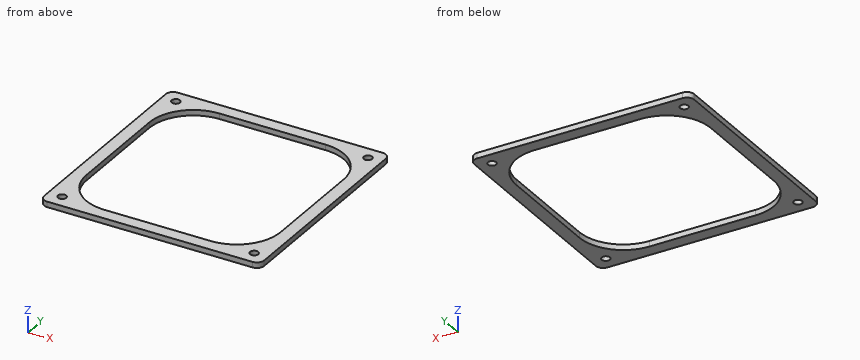
Autodesk Inventor part; units mm, degrees
ref_plane "YZ Plane" through (0, 0, 0) normal (1, 0, 0) x (0, 1, 0)
ref_plane "XZ Plane" through (0, 0, 0) normal (0, 1, 0) x (-1, 0, 0)
ref_plane "XY Plane" through (0, 0, 0) normal (0, 0, 1) x (1, 0, 0)
sketch "スケッチ1" plane through (0, 0, 0) normal (0, 0, 1) x (1, 0, 0)
  circle A0 centre (5, 125) radius 2.25 construction
  circle A1 centre (5, 5) radius 2.25 construction
  circle A2 centre (-473, 125) radius 2.25 construction
  circle A3 centre (-473, 5) radius 2.25 construction
  line L0 (-478, 130) -> (-478, 0) construction
  line L1 (10, 0) -> (10, 130) construction
  line L2 (10, 130) -> (-478, 130)
  line L3 (-478, 130) -> (-478, 0)
  line L4 (-478, 0) -> (10, 0)
  line L5 (10, 0) -> (10, 130)
  circle A4 centre (5, 125) radius 1.6
  circle A5 centre (5, 5) radius 1.6
  circle A6 centre (-473, 5) radius 1.6
  circle A7 centre (-473, 125) radius 1.6
  line L6 (10, 65) -> (-478, 65) construction
  line L7 (-205, 118) -> (-263, 118)
  line L8 (-287, 94) -> (-287, 36)
  line L9 (-263, 12) -> (-205, 12)
  line L10 (-181, 36) -> (-181, 94)
  arc A8 (-181, 94) -> (-205, 118) centre (-205, 94) ccw
  arc A9 (-205, 12) -> (-181, 36) centre (-205, 36) ccw
  arc A10 (-287, 36) -> (-263, 12) centre (-263, 36) ccw
  arc A11 (-263, 118) -> (-287, 94) centre (-263, 94) ccw
  line L11 (-174, 125) -> (-294, 125) construction
  line L12 (-294, 125) -> (-294, 5) construction
  line L13 (-294, 5) -> (-174, 5) construction
  line L14 (-174, 5) -> (-174, 125) construction
  line L15 (-181.6, 117.4) -> (-286.4, 117.4) construction
  line L16 (-286.4, 117.4) -> (-286.4, 12.6) construction
  line L17 (-286.4, 12.6) -> (-181.6, 12.6) construction
  line L18 (-181.6, 12.6) -> (-181.6, 117.4) construction
  circle A12 centre (-181.6, 117.4) radius 2.25
  circle A13 centre (-181.6, 12.6) radius 2.25
  circle A14 centre (-286.4, 12.6) radius 2.25
  circle A15 centre (-286.4, 117.4) radius 2.25
  circle A16 centre (-301.6, 117.4) radius 2.25
  arc A17 (-301, 94) -> (-325, 118) centre (-325, 94) ccw
  line L19 (-301, 36) -> (-301, 94)
  arc A18 (-325, 12) -> (-301, 36) centre (-325, 36) ccw
  circle A19 centre (-301.6, 12.6) radius 2.25
  line L20 (-383, 12) -> (-325, 12)
  arc A20 (-407, 36) -> (-383, 12) centre (-383, 36) ccw
  circle A21 centre (-406.4, 12.6) radius 2.25
  line L21 (-407, 94) -> (-407, 36)
  circle A22 centre (-406.4, 117.4) radius 2.25
  arc A23 (-383, 118) -> (-407, 94) centre (-383, 94) ccw
  line L22 (-325, 118) -> (-383, 118)
  circle A24 centre (-61.6, 117.4) radius 2.25
  arc A25 (-61, 94) -> (-85, 118) centre (-85, 94) ccw
  line L23 (-61, 36) -> (-61, 94)
  arc A26 (-85, 12) -> (-61, 36) centre (-85, 36) ccw
  circle A27 centre (-61.6, 12.6) radius 2.25
  line L24 (-143, 12) -> (-85, 12)
  arc A28 (-167, 36) -> (-143, 12) centre (-143, 36) ccw
  circle A29 centre (-166.4, 12.6) radius 2.25
  line L25 (-167, 94) -> (-167, 36)
  circle A30 centre (-166.4, 117.4) radius 2.25
  arc A31 (-143, 118) -> (-167, 94) centre (-143, 94) ccw
  line L26 (-85, 118) -> (-143, 118)
  circle A32 centre (-181.6, 117.4) radius 2.25
  arc A33 (-181, 94) -> (-205, 118) centre (-205, 94) ccw
  line L27 (-181, 36) -> (-181, 94)
  arc A34 (-205, 12) -> (-181, 36) centre (-205, 36) ccw
  circle A35 centre (-181.6, 12.6) radius 2.25
  line L28 (-263, 12) -> (-205, 12)
  arc A36 (-287, 36) -> (-263, 12) centre (-263, 36) ccw
  circle A37 centre (-286.4, 12.6) radius 2.25
  line L29 (-287, 94) -> (-287, 36)
  circle A38 centre (-286.4, 117.4) radius 2.25
  arc A39 (-263, 118) -> (-287, 94) centre (-263, 94) ccw
  line L30 (-205, 118) -> (-263, 118)
  point P0 (0, 0)
  point P1 (-234, 65)
  point P2 (-287, 12)
  point P3 (-287, 118)
  point P4 (-181, 12)
  point P5 (-287, 65)
  point P6 (-294, 65)
  point P7 (-234, 12)
  point P8 (-234, 5)
  point P9 (-234, 118)
  point P10 (-181, 65)
  point P11 (-174, 65)
  point P12 (-181.6, 65)
  point P13 (-234, 125)
  point P14 (-234, 117.4)
  point P15 (-301, 12)
  point P16 (-301, 65)
  point P17 (-407, 12)
  point P18 (-354, 12)
  point P19 (-407, 118)
  point P20 (-407, 65)
  point P21 (-354, 118)
  point P22 (-61, 12)
  point P23 (-61, 65)
  point P24 (-167, 12)
  point P25 (-114, 12)
  point P26 (-167, 118)
  point P27 (-167, 65)
  point P28 (-114, 118)
  point P29 (-181, 12)
  point P30 (-181, 65)
  point P31 (-287, 12)
  point P32 (-234, 12)
  point P33 (-287, 118)
  point P34 (-287, 65)
  point P35 (-234, 118)
  dimension "d0" = 3.2
  dimension "d1" = 106
  dimension "d2" = 106
  dimension "d3" = 24
  dimension "d4" = 120
  dimension "d5" = 120
  dimension "d6" = 104.8
  dimension "d7" = 104.8
  dimension "d8" = 4.5
  dimension "d11" = 120
  dimension "d14" = 120
extrude "押し出し1" add sketch "スケッチ1" along normal blind 3
sketch "スケッチ2" plane through (0, 0, 3) normal (0, 0, 1) x (1, 0, 0)
  line L0 (-478, 130) -> (-478, 0)
  line L1 (-478, 0) -> (10, 0)
  line L2 (10, 0) -> (10, 130)
  line L3 (10, 130) -> (-478, 130)
  circle A0 centre (-286.4, 117.4) radius 2.25
  arc A1 (-263, 118) -> (-287, 94) centre (-263, 94) ccw
  line L4 (-263, 118) -> (-205, 118)
  arc A2 (-181, 94) -> (-205, 118) centre (-205, 94) ccw
  line L5 (-181, 94) -> (-181, 36)
  arc A3 (-205, 12) -> (-181, 36) centre (-205, 36) ccw
  line L6 (-205, 12) -> (-263, 12)
  arc A4 (-287, 36) -> (-263, 12) centre (-263, 36) ccw
  line L7 (-287, 36) -> (-287, 94)
  circle A5 centre (-473, 125) radius 1.6
  circle A6 centre (-473, 5) radius 1.6
  circle A7 centre (5, 5) radius 1.6
  circle A8 centre (5, 125) radius 1.6
  circle A9 centre (-181.6, 117.4) radius 2.25
  circle A10 centre (-181.6, 12.6) radius 2.25
  circle A11 centre (-286.4, 12.6) radius 2.25
  circle A12 centre (-166.4, 117.4) radius 2.25
  circle A13 centre (-166.4, 12.6) radius 2.25
  circle A14 centre (-61.6, 12.6) radius 2.25
  line L8 (-61, 94) -> (-61, 36)
  arc A15 (-85, 12) -> (-61, 36) centre (-85, 36) ccw
  line L9 (-85, 12) -> (-143, 12)
  arc A16 (-167, 36) -> (-143, 12) centre (-143, 36) ccw
  line L10 (-167, 36) -> (-167, 94)
  arc A17 (-143, 118) -> (-167, 94) centre (-143, 94) ccw
  line L11 (-143, 118) -> (-85, 118)
  arc A18 (-61, 94) -> (-85, 118) centre (-85, 94) ccw
  circle A19 centre (-61.6, 117.4) radius 2.25
  circle A20 centre (-406.4, 117.4) radius 2.25
  circle A21 centre (-406.4, 12.6) radius 2.25
  circle A22 centre (-301.6, 12.6) radius 2.25
  line L12 (-301, 94) -> (-301, 36)
  arc A23 (-325, 12) -> (-301, 36) centre (-325, 36) ccw
  line L13 (-325, 12) -> (-383, 12)
  arc A24 (-407, 36) -> (-383, 12) centre (-383, 36) ccw
  line L14 (-407, 36) -> (-407, 94)
  arc A25 (-383, 118) -> (-407, 94) centre (-383, 94) ccw
  line L15 (-383, 118) -> (-325, 118)
  arc A26 (-301, 94) -> (-325, 118) centre (-325, 94) ccw
  circle A27 centre (-301.6, 117.4) radius 2.25
  line L16 (-477.9, 129.9) -> (-477.9, 0.1)
  line L17 (-477.9, 0.1) -> (9.9, 0.1)
  line L18 (9.9, 0.1) -> (9.9, 129.9)
  line L19 (9.9, 129.9) -> (-477.9, 129.9)
  point P0 (0, 0)
  dimension "d19" = 0.1
extrude "押し出し2" cut sketch "スケッチ2" against normal through all contours L3 L2 L1 L0
fillet "フィレット1" radius 2 4 edges at (-477.9, 129.9, 1.5) (-477.9, 0.1, 1.5) (9.9, 0.1, 1.5) (9.9, 129.9, 1.5)
sketch "スケッチ3" plane through (0, 0, 3) normal (0, 0, 1) x (1, 0, 0)
  arc A0 (9.9, 127.9) -> (7.9, 129.9) centre (7.9, 127.9) ccw
  line L0 (7.9, 129.9) -> (-475.9, 129.9)
  arc A1 (-475.9, 129.9) -> (-477.9, 127.9) centre (-475.9, 127.9) ccw
  line L1 (-477.9, 127.9) -> (-477.9, 2.1)
  arc A2 (-477.9, 2.1) -> (-475.9, 0.1) centre (-475.9, 2.1) ccw
  line L2 (-475.9, 0.1) -> (7.9, 0.1)
  arc A3 (7.9, 0.1) -> (9.9, 2.1) centre (7.9, 2.1) ccw
  line L3 (9.9, 2.1) -> (9.9, 127.9)
  circle A4 centre (-286.4, 117.4) radius 2.25
  arc A5 (-263, 118) -> (-287, 94) centre (-263, 94) ccw
  line L4 (-263, 118) -> (-205, 118)
  arc A6 (-181, 94) -> (-205, 118) centre (-205, 94) ccw
  line L5 (-181, 94) -> (-181, 36)
  arc A7 (-205, 12) -> (-181, 36) centre (-205, 36) ccw
  line L6 (-205, 12) -> (-263, 12)
  arc A8 (-287, 36) -> (-263, 12) centre (-263, 36) ccw
  line L7 (-287, 36) -> (-287, 94)
  circle A9 centre (-473, 125) radius 1.6
  circle A10 centre (-473, 5) radius 1.6
  circle A11 centre (5, 5) radius 1.6
  circle A12 centre (5, 125) radius 1.6
  circle A13 centre (-181.6, 117.4) radius 2.25
  circle A14 centre (-181.6, 12.6) radius 2.25
  circle A15 centre (-286.4, 12.6) radius 2.25
  circle A16 centre (-166.4, 117.4) radius 2.25
  circle A17 centre (-166.4, 12.6) radius 2.25
  circle A18 centre (-61.6, 12.6) radius 2.25
  line L8 (-61, 94) -> (-61, 36)
  arc A19 (-85, 12) -> (-61, 36) centre (-85, 36) ccw
  line L9 (-85, 12) -> (-143, 12)
  arc A20 (-167, 36) -> (-143, 12) centre (-143, 36) ccw
  line L10 (-167, 36) -> (-167, 94)
  arc A21 (-143, 118) -> (-167, 94) centre (-143, 94) ccw
  line L11 (-143, 118) -> (-85, 118)
  arc A22 (-61, 94) -> (-85, 118) centre (-85, 94) ccw
  circle A23 centre (-61.6, 117.4) radius 2.25
  circle A24 centre (-406.4, 117.4) radius 2.25
  circle A25 centre (-406.4, 12.6) radius 2.25
  circle A26 centre (-301.6, 12.6) radius 2.25
  line L12 (-301, 94) -> (-301, 36)
  arc A27 (-325, 12) -> (-301, 36) centre (-325, 36) ccw
  line L13 (-325, 12) -> (-383, 12)
  arc A28 (-407, 36) -> (-383, 12) centre (-383, 36) ccw
  line L14 (-407, 36) -> (-407, 94)
  arc A29 (-383, 118) -> (-407, 94) centre (-383, 94) ccw
  line L15 (-383, 118) -> (-325, 118)
  arc A30 (-301, 94) -> (-325, 118) centre (-325, 94) ccw
  circle A31 centre (-301.6, 117.4) radius 2.25
  line L16 (-410, 125) -> (-58, 125)
  line L17 (-54, 121) -> (-54, 9)
  line L18 (-58, 5) -> (-410, 5)
  line L19 (-414, 9) -> (-414, 121)
  arc A32 (-410, 125) -> (-414, 121) centre (-410, 121) ccw
  arc A33 (-414, 9) -> (-410, 5) centre (-410, 9) ccw
  arc A34 (-58, 5) -> (-54, 9) centre (-58, 9) ccw
  arc A35 (-54, 121) -> (-58, 125) centre (-58, 121) ccw
  line L20 (-294, 125) -> (-294, 5)
  point P0 (0, 0)
  point P1 (-414, 125)
  point P2 (-54, 125)
  point P3 (-234, 125)
  point P4 (-234, 118)
  point P5 (-414, 65)
  point P6 (-407, 65)
  dimension "d23" = 120
  dimension "d24" = 360
  dimension "d25" = 4
  dimension "d28" = 120
extrude "押し出し3" cut sketch "スケッチ3" against normal blind 10 contours A24 | A25 | A26 | A31 | L16 L20 L18 A33 L19 A32 keep common part
fillet "フィレット2" radius 4 2 edges at (-294, 125, 1.5) (-294, 5, 1.5)
equation "\"d5\" = d4"
equation "\"d7\" = d6"
properties part number "radiator_adapter_04"
The listing builds one solid part. Answer for the finished solid, in the listing's coordinates (mm). Give positions to 0.01 mm unless a question says otherwise; leave off trailing zeros. Write each loop counter-clockwise with the first axis right and the second up, starting at its lowest first coordinate (ties: lowest second). Pieces come first, ordered by that corner, then holes. Notation, with made-up numbers: (79, 32) - (136, 32) arc R20 cw to (136, 51) - close; hole circle Ø11 at (46.25, 46). An arc over 180 degrees is marked (long way). Use one line per item in the form item = value. Start each with the question number.
1) Find section C-C on z = 2.1. Determine the outline of the cut face in (x, y), plus the area to 3 significant figures.
2) Find section A-A on x = -343. Determine the outline of the cut face in (y, z).
3) Find section B-B on y = 91. Determine the outline of the cut face in (x, z), plus the area to 3 significant figures.
4) Consider line 1 along Y through (x, z) = (-353, 1.1); line 2 along X through (y, z) = (45, 1); line 3 along X through (y, z) = (105, 1.1). Determine where each line is inside the solid, lowest interval first. Write a range as from..to.
Geometry results:
q1.outline = (-414, 9) arc R4 ccw to (-410, 5) - (-298, 5) arc R4 ccw to (-294, 9) - (-294, 121) arc R4 ccw to (-298, 125) - (-410, 125) arc R4 ccw to (-414, 121) - close; hole circle Ø4.5 at (-406.4, 12.6); hole circle Ø4.5 at (-406.4, 117.4); hole (-407, 36) arc R24 ccw to (-383, 12) - (-325, 12) arc R24 ccw to (-301, 36) - (-301, 94) arc R24 ccw to (-325, 118) - (-383, 118) arc R24 ccw to (-407, 94) - close; hole circle Ø4.5 at (-301.6, 12.6); hole circle Ø4.5 at (-301.6, 117.4)
q1.area = 3,580 mm2
q2.outline = (5, 0) - (12, 0) - (12, 3) - (5, 3) - close; (118, 0) - (125, 0) - (125, 3) - (118, 3) - close
q3.outline = (-414, 0) - (-407, 0) - (-407, 3) - (-414, 3) - close; (-301, 0) - (-294, 0) - (-294, 3) - (-301, 3) - close
q3.area = 42.0 mm2
q4.line_1 = 5..12, 118..125
q4.line_2 = -414..-407, -301..-294
q4.line_3 = -414..-404.33, -303.67..-294
